Input: dimensioned drawing with shaded views. Units: mm. Origin: part minimum x, y, z. A direction names the side the tool comes from. Round coordinates to 2 decimals unless told otherwise and drop trailing zeros. Order: outer loops, then holes, each group sorted by start corner. A loop starts at its lowest first (then second) coordinate and runs counter-clockwise, first axis right, second up. Notation, with made-up numbers: M 69.25,-29 L 120.25,-29 A33 cw 120.25,6 Z; hole C 37,-17 d2. An arc over 180 degrees is marked long. Use one line per item in the form item = value. Start each with the question number.
Q1. Material intervals for probe 1 along Z at (x, y) = (9, 8); probe 2 along Y at (x, z) = (48, 4.5) (1 decimal); probe 3 along Y at (x, z) = (15, 4), sorted ascending.
Q2. Section C-C (x = 25). Return the cut outline in (y, z), plus the area to 3 significant figures.
Q3. Section A-A (y = 25). Return the cut outline in (x, z), plus the area to 3 significant figures.
Q4. Contact query for flat-ended pins moving along their axis: pin 1 (8 mm diameter, centred on x = 30, z = 12, fed in from -Y); pin 2 (8 mm diameter, centred on y = 21, z = 6, fed in from -X); pin 3 (4 mm diameter, centred on x = 10, z = 33.5, fed in from -Y); pin 4 (2 mm diameter, centred on x = 33.5, z = 39, fed in from +Y). Output: stop coordinate, or through.
Q5. Section B-B (z = 41). Return the cut outline in (x, y).
Q6. Section D-D (y = 40). Return the cut outline in (x, z), plus the area to 3 significant figures.
Q7. Reachability of the marked faces 1 and 2 from +Z, -Z, +X, -X, +Y, -Y: full face, straight path, thin tool, end or side. Return the list, or none.
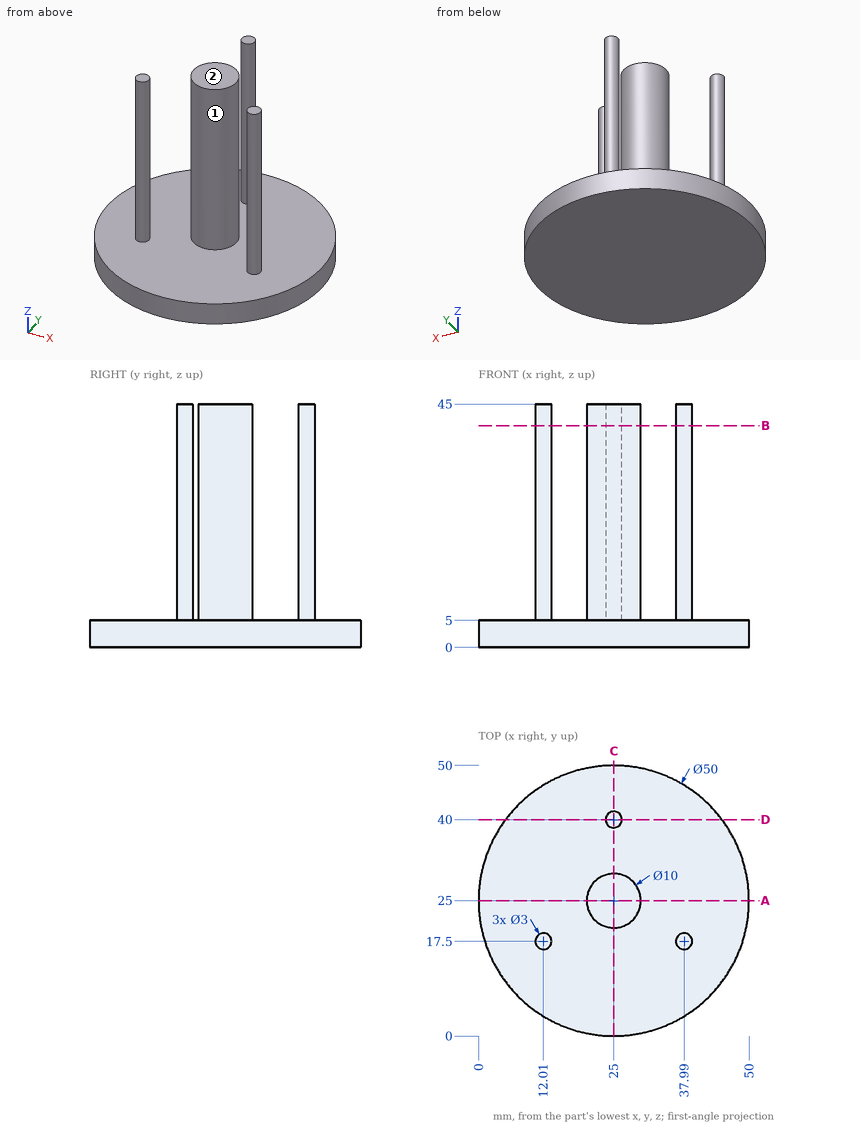
Results list:
q1.probe_1 = 0 to 5
q1.probe_2 = 15.2 to 34.8
q1.probe_3 = 2.09 to 47.91
q2.outline = M 0,0 L 50,0 L 50,5 L 41.5,5 L 41.5,45 L 38.5,45 L 38.5,5 L 30,5 L 30,45 L 20,45 L 20,5 L 0,5 Z
q2.area = 770 mm2
q3.outline = M 0,0 L 50,0 L 50,5 L 30,5 L 30,45 L 20,45 L 20,5 L 0,5 Z
q3.area = 650 mm2
q4.pin_1 = 20.1
q4.pin_2 = 0
q4.pin_3 = 16
q4.pin_4 = through
q5.outline = C 12.01,17.5 d3; C 25,25 d10; C 25,40 d3; C 37.99,17.5 d3
q6.outline = M 5,0 L 45,0 L 45,5 L 26.5,5 L 26.5,45 L 23.5,45 L 23.5,5 L 5,5 Z
q6.area = 320 mm2
q7.face_1 = +Z
q7.face_2 = +Z, +X, -X, +Y, -Y
